Read the model definition and answer for the solid it produces. Units are mm, in the model's axes. Coordinates: 2 decimals unless noted, no trailing zeros. Order: outer loops, then holes, each group sorted by start corner. A loop starts at its lowest first (then second) coordinate and runs counter-clockwise, first axis right, second up.
```python
from build123d import *

# Parameters (mm, degrees)
F0_R     = 0.5
F1_DEPTH = 1
F2_DEPTH = 15
F3_DEPTH = 3


with BuildPart() as f1:
    # F0 (on Front) → F1 (new body)
    with BuildSketch(Plane.XZ):
        with BuildLine():
            ThreePointArc((-6.244998, 0.25), (-4.419417, 4.419417), (-0.25, 6.244998))
            Line((-0.25, 6.244998), (-0.282, 7.044358))
            ThreePointArc((-0.282, 7.044358), (-4.985103, 4.985103), (-7.044358, 0.282))
            Line((-7.044358, 0.282), (-6.244998, 0.25))
        make_face()
        with BuildLine():
            ThreePointArc((-0.25, 6.244998), (0, 6.25), (0.25, 6.244998))
            Line((0.25, 6.244998), (0.282, 7.044358))
            ThreePointArc((0.282, 7.044358), (0, 7.05), (-0.282, 7.044358))
            Line((-0.282, 7.044358), (-0.25, 6.244998))
        make_face()
        with BuildLine():
            ThreePointArc((6.25, 0), (6.248749, 0.125025), (6.244998, 0.25))
            ThreePointArc((6.244998, 0.25), (4.419417, 4.419417), (0.25, 6.244998))
            ThreePointArc((0.25, 6.244998), (0, 6.25), (-0.25, 6.244998))
            ThreePointArc((-0.25, 6.244998), (-4.419417, 4.419417), (-6.244998, 0.25))
            ThreePointArc((-6.244998, 0.25), (-6.25, 0), (-6.244998, -0.25))
            ThreePointArc((-6.244998, -0.25), (-4.419417, -4.419417), (-0.25, -6.244998))
            ThreePointArc((-0.25, -6.244998), (0, -6.25), (0.25, -6.244998))
            ThreePointArc((0.25, -6.244998), (4.419417, -4.419417), (6.244998, -0.25))
            ThreePointArc((6.244998, -0.25), (6.248749, -0.125025), (6.25, 0))
        make_face()
        with Locations((-2.12132, -2.12132)):
            Circle(F0_R, mode=Mode.SUBTRACT)
        with Locations((2.12132, -2.12132)):
            Circle(F0_R, mode=Mode.SUBTRACT)
        with Locations((-2.12132, 2.12132)):
            Circle(F0_R, mode=Mode.SUBTRACT)
        with Locations((2.12132, 2.12132)):
            Circle(F0_R, mode=Mode.SUBTRACT)
        with BuildLine():
            ThreePointArc((0.25, 6.244998), (4.419417, 4.419417), (6.244998, 0.25))
            Line((6.244998, 0.25), (7.044358, 0.282))
            ThreePointArc((7.044358, 0.282), (4.985103, 4.985103), (0.282, 7.044358))
            Line((0.282, 7.044358), (0.25, 6.244998))
        make_face()
        with BuildLine():
            Line((7.044358, 0.282), (6.244998, 0.25))
            ThreePointArc((6.244998, 0.25), (6.248749, 0.125025), (6.25, 0))
            ThreePointArc((6.25, 0), (6.248749, -0.125025), (6.244998, -0.25))
            Line((6.244998, -0.25), (7.044358, -0.282))
            ThreePointArc((7.044358, -0.282), (7.048589, -0.141028), (7.05, 0))
            ThreePointArc((7.05, 0), (7.048589, 0.141028), (7.044358, 0.282))
        make_face()
        with BuildLine():
            Line((7.044358, -0.282), (6.244998, -0.25))
            ThreePointArc((6.244998, -0.25), (4.419417, -4.419417), (0.25, -6.244998))
            Line((0.25, -6.244998), (0.282, -7.044358))
            ThreePointArc((0.282, -7.044358), (4.985103, -4.985103), (7.044358, -0.282))
        make_face()
        with BuildLine():
            Line((0.282, -7.044358), (0.25, -6.244998))
            ThreePointArc((0.25, -6.244998), (0, -6.25), (-0.25, -6.244998))
            Line((-0.25, -6.244998), (-0.282, -7.044358))
            ThreePointArc((-0.282, -7.044358), (0, -7.05), (0.282, -7.044358))
        make_face()
        with BuildLine():
            ThreePointArc((-0.25, -6.244998), (-4.419417, -4.419417), (-6.244998, -0.25))
            Line((-6.244998, -0.25), (-7.044358, -0.282))
            ThreePointArc((-7.044358, -0.282), (-4.985103, -4.985103), (-0.282, -7.044358))
            Line((-0.282, -7.044358), (-0.25, -6.244998))
        make_face()
        with BuildLine():
            ThreePointArc((-6.244998, -0.25), (-6.25, 0), (-6.244998, 0.25))
            Line((-6.244998, 0.25), (-7.044358, 0.282))
            ThreePointArc((-7.044358, 0.282), (-7.05, 0), (-7.044358, -0.282))
            Line((-7.044358, -0.282), (-6.244998, -0.25))
        make_face()
    extrude(amount=-F1_DEPTH)

    # F0 (on Front) → F2 (join)
    with BuildSketch(Plane.XZ):
        with BuildLine():
            ThreePointArc((-6.244998, 0.25), (-4.419417, 4.419417), (-0.25, 6.244998))
            Line((-0.25, 6.244998), (-0.282, 7.044358))
            ThreePointArc((-0.282, 7.044358), (-4.985103, 4.985103), (-7.044358, 0.282))
            Line((-7.044358, 0.282), (-6.244998, 0.25))
        make_face()
        with BuildLine():
            ThreePointArc((0.25, 6.244998), (4.419417, 4.419417), (6.244998, 0.25))
            Line((6.244998, 0.25), (7.044358, 0.282))
            ThreePointArc((7.044358, 0.282), (4.985103, 4.985103), (0.282, 7.044358))
            Line((0.282, 7.044358), (0.25, 6.244998))
        make_face()
        with BuildLine():
            Line((7.044358, -0.282), (6.244998, -0.25))
            ThreePointArc((6.244998, -0.25), (4.419417, -4.419417), (0.25, -6.244998))
            Line((0.25, -6.244998), (0.282, -7.044358))
            ThreePointArc((0.282, -7.044358), (4.985103, -4.985103), (7.044358, -0.282))
        make_face()
        with BuildLine():
            ThreePointArc((-0.25, -6.244998), (-4.419417, -4.419417), (-6.244998, -0.25))
            Line((-6.244998, -0.25), (-7.044358, -0.282))
            ThreePointArc((-7.044358, -0.282), (-4.985103, -4.985103), (-0.282, -7.044358))
            Line((-0.282, -7.044358), (-0.25, -6.244998))
        make_face()
    extrude(amount=F2_DEPTH)

    # F0 (on Front) → F3 (join)
    with BuildSketch(Plane.XZ):
        with BuildLine():
            ThreePointArc((-6.244998, -0.25), (-6.25, 0), (-6.244998, 0.25))
            Line((-6.244998, 0.25), (-7.044358, 0.282))
            ThreePointArc((-7.044358, 0.282), (-7.05, 0), (-7.044358, -0.282))
            Line((-7.044358, -0.282), (-6.244998, -0.25))
        make_face()
        with BuildLine():
            Line((0.282, -7.044358), (0.25, -6.244998))
            ThreePointArc((0.25, -6.244998), (0, -6.25), (-0.25, -6.244998))
            Line((-0.25, -6.244998), (-0.282, -7.044358))
            ThreePointArc((-0.282, -7.044358), (0, -7.05), (0.282, -7.044358))
        make_face()
        with BuildLine():
            Line((7.044358, 0.282), (6.244998, 0.25))
            ThreePointArc((6.244998, 0.25), (6.248749, 0.125025), (6.25, 0))
            ThreePointArc((6.25, 0), (6.248749, -0.125025), (6.244998, -0.25))
            Line((6.244998, -0.25), (7.044358, -0.282))
            ThreePointArc((7.044358, -0.282), (7.048589, -0.141028), (7.05, 0))
            ThreePointArc((7.05, 0), (7.048589, 0.141028), (7.044358, 0.282))
        make_face()
        with BuildLine():
            ThreePointArc((-0.25, 6.244998), (0, 6.25), (0.25, 6.244998))
            Line((0.25, 6.244998), (0.282, 7.044358))
            ThreePointArc((0.282, 7.044358), (0, 7.05), (-0.282, 7.044358))
            Line((-0.282, 7.044358), (-0.25, 6.244998))
        make_face()
    extrude(amount=F3_DEPTH)


solid = f1.part
```
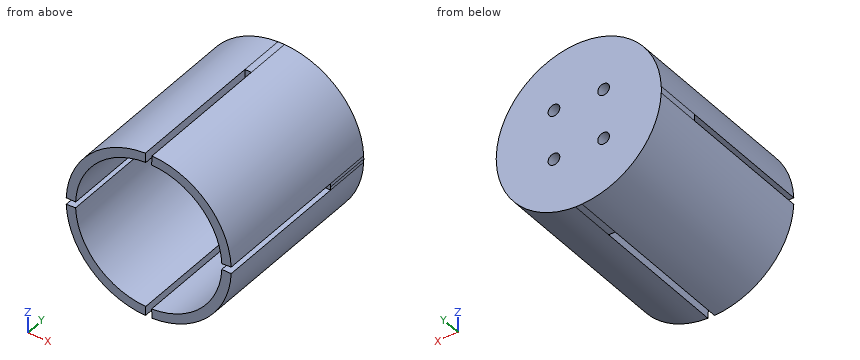
1) A cutting plane is placed at C-C, the plane x = 4.5. Determine the outline of the cut face in (y, z), and give its area (3 significant figures).
A:
outline: (-15, -5.43) - (1, -5.43) - (1, 5.43) - (-15, 5.43) - (-15, 4.34) - (0, 4.34) - (0, -4.34) - (-15, -4.34) - close
area: 43.5 mm2
2) A cutting plane is placed at B-B, the plane y = -1. Determine the outline of the cut face in (x, z) (3 decimals).
A:
outline: (-7.044, -0.282) arc R7.05 ccw to (-0.282, -7.044) arc R7.05 ccw to (0.282, -7.044) arc R7.05 ccw to (7.044, -0.282) arc R7.052 ccw to (7.05, 0) arc R7.052 ccw to (7.044, 0.282) arc R7.05 ccw to (0.282, 7.044) arc R7.05 ccw to (-0.282, 7.044) arc R7.05 ccw to (-7.044, 0.282) arc R7.05 ccw to start; hole (-6.245, -0.25) arc R6.25 ccw to (-0.25, -6.245) arc R6.25 ccw to (0.25, -6.245) arc R6.25 ccw to (6.245, -0.25) arc R6.252 ccw to (6.25, 0) arc R6.252 ccw to (6.245, 0.25) arc R6.25 ccw to (0.25, 6.245) arc R6.25 ccw to (-0.25, 6.245) arc R6.25 ccw to (-6.245, 0.25) arc R6.25 ccw to start
3) A cutting plane is placed at A-A, the plane y = -11.5. Determine the outline of the cut face in (x, z) (3 decimals).
A:
outline: (-7.044, -0.282) arc R7.05 ccw to (-0.282, -7.044) - (-0.25, -6.245) arc R6.25 cw to (-6.245, -0.25) - close; (-7.044, 0.282) - (-6.245, 0.25) arc R6.25 cw to (-0.25, 6.245) - (-0.282, 7.044) arc R7.05 ccw to start; (0.25, -6.245) - (0.282, -7.044) arc R7.05 ccw to (7.044, -0.282) - (6.245, -0.25) arc R6.25 cw to start; (0.25, 6.245) arc R6.25 cw to (6.245, 0.25) - (7.044, 0.282) arc R7.05 ccw to (0.282, 7.044) - close
4) A cutting plane is placed at D-D, the plane z = 4.5. Determine the outline of the cut face in (x, y), and give its area (3 significant figures).
A:
outline: (-5.43, -15) - (-4.34, -15) - (-4.34, 0) - (4.34, 0) - (4.34, -15) - (5.43, -15) - (5.43, 1) - (-5.43, 1) - close
area: 43.5 mm2
5) Straight lines are drawn through the part: line 1 (X direction, y = 0.25, z = -2.5); line 2 (Y direction, x = -5.75, z = -1.5); line 3 (Z direction, x = 1.5, y = -10.5). For each, find the intervals that lie inside material, in ascending order.
A:
line 1: x = -6.59 to -2.45, -1.79 to 1.79, 2.45 to 6.59
line 2: y = 0 to 1
line 3: z = -6.89 to -6.07, 6.07 to 6.89
6) Flat-ended cylindrical pins translate along their axes: pin 1 Ø8 at (x, z) = (-4, -3.5) entering from -Y; pin 2 Ø6 at (x, y) = (-2.5, -6.5) entering from +Z; pin 3 Ø2 at (x, y) = (-4.5, -1) entering from +Z; pin 4 Ø2 at (x, z) = (-0.5, 4.5) entering from -Y. Find the tip coordinate at first contact, or state that the pin passes through.
A:
pin 1: stops at y = -15
pin 2: stops at z = 7.04
pin 3: stops at z = 6.12
pin 4: stops at y = 0
